from build123d import *

# Parameters (mm, degrees)
SKETCH1_W           = 190
SKETCH1_H           = 112
BOSS_EXTRUDE1_DEPTH = 15
SKETCH5_W           = 102
SKETCH5_H           = 12
CUT_EXTRUDE3_DEPTH  = 222.06333934
CUT_EXTRUDE4_DEPTH  = 10
SKETCH6_R           = 3
CUT_EXTRUDE5_DEPTH  = 10


with BuildPart() as part:
    # Sketch1 → Boss-Extrude1 (new body)
    with BuildSketch(Plane(origin=(0, 0, 0), x_dir=(1, 0, 0), z_dir=(0, 1, 0))):
        with Locations((95, -56)):
            Rectangle(SKETCH1_W, SKETCH1_H)
    extrude(amount=BOSS_EXTRUDE1_DEPTH)

    # Sketch5 → Cut-Extrude3 (cut, through all)
    with BuildSketch(Plane(origin=(190, 0, 0), x_dir=(0, 0, -1), z_dir=(1, 0, 0))):
        with Locations((-56, 6)):
            Rectangle(SKETCH5_W, SKETCH5_H)
    extrude(amount=-CUT_EXTRUDE3_DEPTH, mode=Mode.SUBTRACT)

    # Sketch2 → Cut-Extrude4 (cut)
    with BuildSketch(Plane.XY.offset(112)):
        with BuildLine():
            Line((34, 10), (156, 10))
            ThreePointArc((156, 10), (159, 7), (156, 4))
            Line((156, 4), (34, 4))
            ThreePointArc((34, 4), (31, 7), (34, 10))
        make_face()
    extrude(amount=-CUT_EXTRUDE4_DEPTH, mode=Mode.SUBTRACT)

    # Sketch6 → Cut-Extrude5 (cut)
    with BuildSketch(Plane(origin=(0, 0, 0), x_dir=(-1, 0, 0), z_dir=(0, 0, -1))):
        with Locations((-95, 7.5)):
            Circle(SKETCH6_R)
    extrude(amount=-CUT_EXTRUDE5_DEPTH, mode=Mode.SUBTRACT)


solid = part.part
CAD build for the part. Positions are in the model's coordinates, mm. A direction names the side the tool comes from. Give positions to 0.01 mm unless a question says otherwise; leave off trailing zeros. Order: outer loops, then holes, each group sorted by start corner. A loop starts at its lowest first (then second) coordinate and runs counter-clockwise, first axis right, second up. Notation, with made-up numbers: (6.5, -12) - (39.5, -12) arc R20 cw to (39.5, 3) - close; hole circle Ø10 at (-38.75, -17.75). An arc over 180 degrees is marked (long way). Answer in a Markdown table with one row per item.
1. Pull direction Y, two halves, no side cores. Call faces 1 (the flat face through (94, 11, 112)), 2 (the flat face through (94, 0, 2)), 3 (the cylindrical face through (31, 7, 110)): pulls with the +Y half, pulls with the -Y half, needs draft (parallel to the pull), parting line crosses it, or undercut.
Data:
| item | result |
|---|---|
| face 1 | needs draft |
| face 2 | pulls with the -Y half |
| face 3 | undercut |
2. Tool access for faces 4 (the flat face through (96, 12, 57)), 5 (the cylindrical face through (159, 7, 110)), 6 (the cylindrical face through (98, 7.6, 2.5)), 7 (the flat face through (94, 0, 109)): list every direction of +Z, -Z, +X, -X, +Y, -Y with a clear straight run to the whole face (end or side of a thin tool).
Data:
| item | result |
|---|---|
| face 4 | +X, -X, -Y |
| face 5 | +Z |
| face 6 | -Z |
| face 7 | +Z, -Z, +X, -X, -Y |
3. Saw through at A-A, the plane x = 118.5. Give the cut face in (y, z), plus the area to 3 significant figures.
Data:
| item | result |
|---|---|
| outline | (0, 0) - (15, 0) - (15, 112) - (10, 112) - (10, 107) - (12, 107) - (12, 5) - (0, 5) - close; (0, 107) - (4, 107) - (4, 112) - (0, 112) - close |
| area | 426 mm² |
4. Saw through at B-B, the plane y = 7.5. Give the cut face in (x, z).
Data:
| item | result |
|---|---|
| outline | (0, 0) - (92, 0) - (92, 5) - (0, 5) - close; (0, 107) - (31.04, 107) - (31.04, 112) - (0, 112) - close; (98, 0) - (190, 0) - (190, 5) - (98, 5) - close; (158.96, 107) - (190, 107) - (190, 112) - (158.96, 112) - close |
5. Probe probe 1 along Y at (x, z) = (95, 2.1); probe 2 along Z at (x, y) = (178.5, 0.75); probe 3 along Y at (x, z) = (164.5, 37.5). List the from-to ranges inside material, lowest first. Write a range as [from, to].
Data:
| item | result |
|---|---|
| probe 1 | y = [0, 4.5], [10.5, 15] |
| probe 2 | z = [0, 5], [107, 112] |
| probe 3 | y = [12, 15] |
6. Saw through at D-D, the plane x = 13.5. Give the cut face in (y, z), plus the area to 3 significant figures.
Data:
| item | result |
|---|---|
| outline | (0, 0) - (15, 0) - (15, 112) - (0, 112) - (0, 107) - (12, 107) - (12, 5) - (0, 5) - close |
| area | 456 mm² |
7. Saw through at C-C, the plane x = 95. Give the cut face in (y, z), plus the area to 3 significant figures.
Data:
| item | result |
|---|---|
| outline | (0, 0) - (4.5, 0) - (4.5, 5) - (0, 5) - close; (0, 107) - (4, 107) - (4, 112) - (0, 112) - close; (10, 107) - (12, 107) - (12, 5) - (10.5, 5) - (10.5, 0) - (15, 0) - (15, 112) - (10, 112) - close |
| area | 396 mm² |
8. Flat gauge pin, fed straight in: pin 1 (6 mm diameter, centred on x = 80.5, z = 15, fed in from -Y). Where does the tip first touch, or does it go through?
Data:
| item | result |
|---|---|
| pin 1 | stops at y = 12 |
